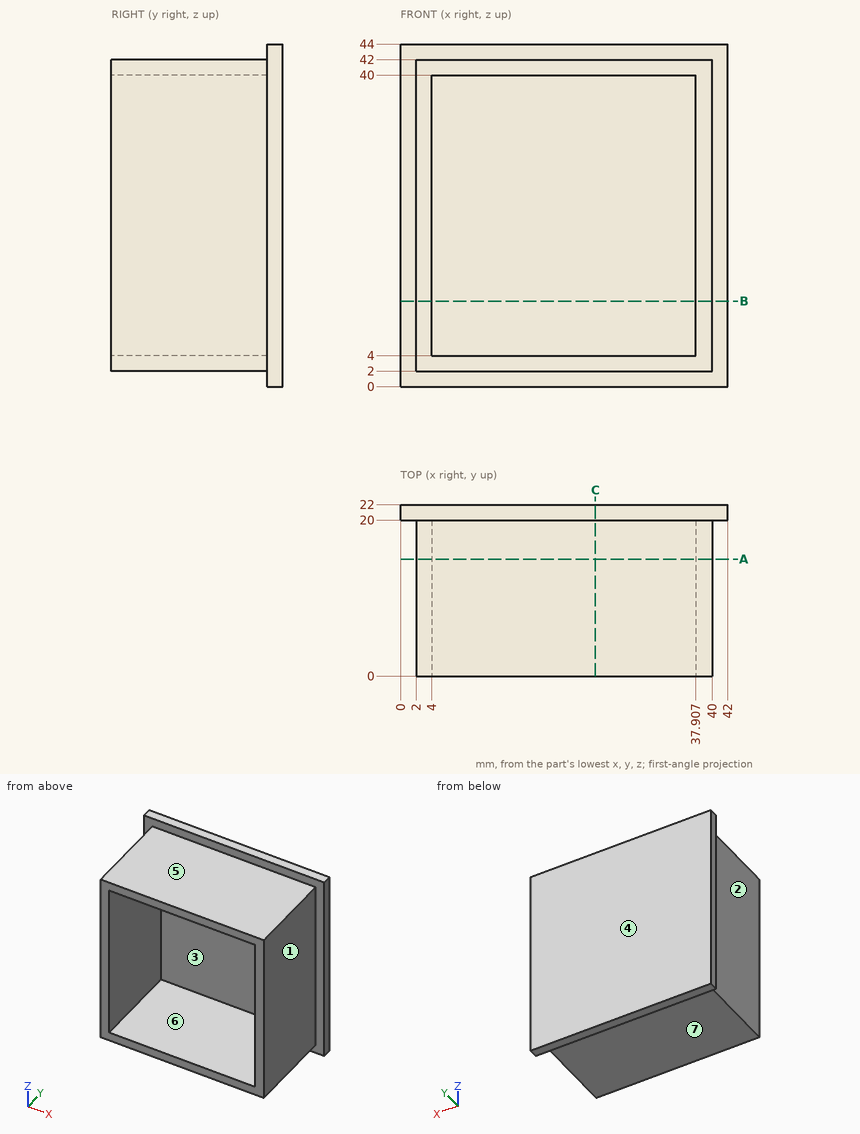
Job drawing, mm, ordinate dimensions from the low corner. One solid piece. A direction names the side the tool comes from. Give positions to 0.01 mm unless a question says otherwise; leave off trailing zeros. Loops run counter-clockwise (first coordinate to the right, second up) from the corner with the lowest first, then second, coordinate; pieces in that order, holes last. Notation, with made-up numbers: (86, 36) -> (116, 36) arc R25 cw to (116, 62) -> close; hole circle Ø7 at (13.25, -1.5). An arc over 180 degrees is marked (long way). Use a Markdown table: item, result. Add a question column.
(1) Tool access for the marked faces 1, 2, 3 and 4: list every direction of +Z, -Z, +X, -X, +Y, -Y with a clear straight run to the whole face (end or side of a thin tool).
(2) Drop flat-ended pins along their axis: pin 1 Ø1 at (x, y) = (27.5, 5.5) entering from -Z; pin 2 Ø10 at (y, z) = (13, 15) entering from +X; pin 3 Ø2 at (x, y) = (7, 5) entering from +Z. Give the stop position or say it passes through.
(3) Slice it at B-B on z = 11. List the corners of the cut face in (x, y), and give its area (3 significant figures).
(4) Slice it at C-C on x = 25. List the corners of the cut face in (y, z), and give its area (3 significant figures).
(5) Wall check: line 1 along Z through (x, y) = (22, 15.25); line 2 along X through (y, z) = (8.5, 9); line 3 along Y through (x, z) = (32.5, 39). Give the ranges that are in metal, low to high.
(6) Mould opens along Z. For the marked faces 5, 6 and 7 say: +Z half, -Z half, draft (parallel to the pull), parting line (faces both ways), or undercut.
(7) Slice it at A-A on y = 15. List the corners of the cut face in (x, z).
Filled sheet:
| question | item | result |
|---|---|---|
| 1 | face 1 | +Z, -Z, +X, -Y |
| 1 | face 2 | +Z, -Z, -X, -Y |
| 1 | face 3 | -Y |
| 1 | face 4 | +Z, -Z, +X, -X, +Y |
| 2 | pin 1 | z = 2 |
| 2 | pin 2 | x = 40 |
| 2 | pin 3 | z = 42 |
| 3 | outline | (0, 20) -> (2, 20) -> (2, 0) -> (4, 0) -> (4, 20) -> (37.91, 20) -> (37.91, 0) -> (40, 0) -> (40, 20) -> (42, 20) -> (42, 22) -> (0, 22) -> close |
| 3 | area | 166 mm2 |
| 4 | outline | (0, 2) -> (20, 2) -> (20, 0) -> (22, 0) -> (22, 44) -> (20, 44) -> (20, 42) -> (0, 42) -> (0, 40) -> (20, 40) -> (20, 4) -> (0, 4) -> close |
| 4 | area | 168 mm2 |
| 5 | line 1 | 2 to 4, 40 to 42 |
| 5 | line 2 | 2 to 4, 37.91 to 40 |
| 5 | line 3 | 20 to 22 |
| 6 | face 5 | +Z half |
| 6 | face 6 | undercut |
| 6 | face 7 | -Z half |
| 7 | outline | (2, 2) -> (40, 2) -> (40, 42) -> (2, 42) -> close; hole (4, 4) -> (37.91, 4) -> (37.91, 40) -> (4, 40) -> close |
